Can you work these out from the model? Positions are in its coordinate system, mm. Face numbers are marked on the shaded views. A direction names the side the tool comes from. Round coordinates to 2 decimals unless told otherwise and drop trailing zeros. Order: outer loops, then holes, each group sorted by start corner. A loop starts at its lowest first (then second) coordinate and runs counter-clockwise, first axis right, second up. Notation, with made-up numbers: M 77,19.25 L 94,19.25 A16 cw 94,38.25 Z; hole C 70,-13.5 d8. An arc over 180 degrees is marked long. One line per question, with ' | ' between items.
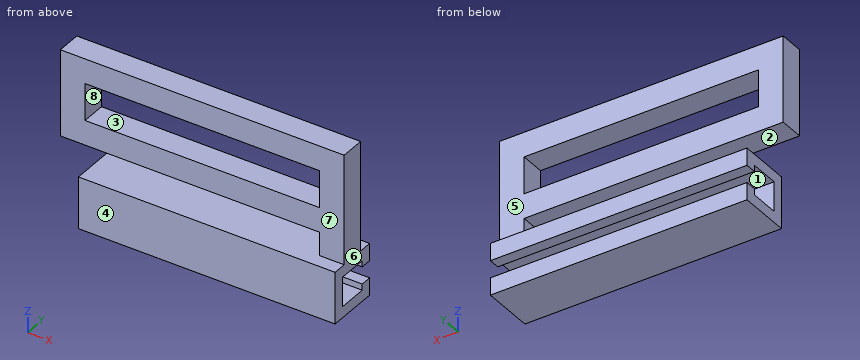
```python
from build123d import *

# Parameters (mm, degrees)
ESBO_O1_W                = 19
ESBO_O1_H                = 3
RESSALTO_EXTRUS_O1_DEPTH = 2
ESBO_O3_W                = 2.338389472
ESBO_O3_H                = 3.565642473
CORTE_EXTRUS_O2_DEPTH    = 3
ESBO_O4_W                = 4.2
ESBO_O4_H                = 4.2
ESBO_O4_W_2              = 2.2
ESBO_O4_H_2              = 2.2
RESSALTO_EXTRUS_O2_DEPTH = 21
ESBO_O5_W                = 2
ESBO_O5_H                = 2
CORTE_EXTRUS_O3_DEPTH    = 29
ESBO_O6_W                = 10.73629406
ESBO_O6_H                = 11.045994849
CORTE_EXTRUS_O4_DEPTH    = 4.5
CORTE_EXTRUS_O5_DEPTH    = 24


with BuildPart() as part:
    # Esboço1 → Ressalto-extrusão1 (new body)
    with BuildSketch(Plane(origin=(0, 0, 0), x_dir=(1, 0, 0), z_dir=(0, 1, 0))):
        Polygon((-10.479474548, 11.375), (12.520525452, 11.375), (12.520525452, -0.625), (10.520525452, -0.625), (-10.479474548, -0.625), (-10.479474548, 6.375), (10.520525452, 6.375), (10.520525452, 9.375), (-10.479474548, 9.375), align=None)
        with Locations((1.020525452, 2.875)):
            Rectangle(ESBO_O1_W, ESBO_O1_H, mode=Mode.SUBTRACT)
    extrude(amount=RESSALTO_EXTRUS_O1_DEPTH)

    # Esboço3 → Corte-extrusão2 (cut)
    with BuildSketch(Plane(origin=(0, 0, 0), x_dir=(1, 0, 0), z_dir=(0, 1, 0))):
        with Locations((-9.648669284, 10.261118249)):
            Rectangle(ESBO_O3_W, ESBO_O3_H)
    extrude(amount=CORTE_EXTRUS_O2_DEPTH, mode=Mode.SUBTRACT)

    # Esboço4 → Ressalto-extrusão2 (add)
    with BuildSketch(Plane.ZY.offset(8.479474548)):
        with Locations((-10.375, 1)):
            Rectangle(ESBO_O4_W, ESBO_O4_H)
        with Locations((-10.375, 1)):
            Rectangle(ESBO_O4_W_2, ESBO_O4_H_2, mode=Mode.SUBTRACT)
    extrude(amount=-RESSALTO_EXTRUS_O2_DEPTH)

    # Esboço5 → Corte-extrusão3 (cut)
    with BuildSketch(Plane.ZY.offset(8.479474548)):
        with Locations((-10.375, 1)):
            Rectangle(ESBO_O5_W, ESBO_O5_H)
    extrude(amount=-CORTE_EXTRUS_O3_DEPTH, mode=Mode.SUBTRACT)

    # Esboço6 → Corte-extrusão4 (cut, symmetric)
    with BuildSketch(Plane(origin=(0, 0, 0), x_dir=(1, 0, 0), z_dir=(0, 1, 0))):
        with Locations((-13.647621578, 13.152356314)):
            Rectangle(ESBO_O6_W, ESBO_O6_H)
    extrude(amount=CORTE_EXTRUS_O4_DEPTH, both=True, mode=Mode.SUBTRACT)

    # Esboço7 → Corte-extrusão5 (cut)
    with BuildSketch(Plane.ZY.offset(8.279474548)):
        Polygon((-11.075, 2.2), (-11.075, 3.370047827), (-9.675, 3.370047827), (-9.675, 2.2), (-9.175, 2.2), (-9.175, -0.2), (-11.575, -0.2), (-11.575, 2.2), align=None)
    extrude(amount=-CORTE_EXTRUS_O5_DEPTH, mode=Mode.SUBTRACT)


solid = part.part
```
(1) If we section it at D-D on y = 2.5: Please give me the cut outline in (x, z) (3 decimals), plus the area to 3 significant figures.
Final values:
outline: M -8.279,-12.475 L 12.521,-12.475 L 12.521,-11.075 L -8.279,-11.075 Z; M -8.279,-9.675 L 12.521,-9.675 L 12.521,-8.275 L -8.279,-8.275 Z | area: 58.2 mm^2
(2) On a 3-axis mill with a long thin cutter (end or side, diameter ignored), from which of +Z, -Z, +X, -X, +Y, -Y can I reach the whole of each face in a straight line? I mean the marked faces 1, 2, 3, 4 and 5. Say none if no direction works.
Final values:
face 1: +X, -X | face 2: -X, +Y, -Y | face 3: +Y, -Y | face 4: +Z, -Z, +X, -X, -Y | face 5: +Z, +X, -X, +Y
(3) If we section it at A-A on y = 1.55: Please give me the cut outline in (x, z) (3 decimals), plus the area to 3 significant figures.
Final values:
outline: M -10.479,-6.375 L 10.521,-6.375 L 10.521,-8.275 L -8.279,-8.275 L -8.279,-9.175 L 12.521,-9.175 L 12.521,0.625 L -10.479,0.625 Z; M -8.279,-12.475 L 12.521,-12.475 L 12.521,-11.575 L -8.279,-11.575 Z; hole M -8.479,-4.375 L 10.521,-4.375 L 10.521,-1.375 L -8.479,-1.375 Z | area: 145 mm^2
(4) If we section it at C-C on z = -2.75: Please give me the cut outline in (x, y), plus the area to 3 significant figures.
Final values:
outline: M -10.48,0 L -8.48,0 L -8.48,2 L -10.48,2 Z; M 10.52,0 L 12.52,0 L 12.52,2 L 10.52,2 Z | area: 8.00 mm^2
(5) Please list where these lines run through material, in increasing order: probe 1 along Z at (x, y) = (6.25, 1.2) (3 decimals); probe 2 along Y at (x, z) = (5.5, -11.25); probe 3 along Z at (x, y) = (9, 2.1) (3 decimals). Write a range as [from, to].
Final values:
probe 1: [-12.475, -11.575], [-9.175, -8.275], [-6.375, -4.375], [-1.375, 0.625] | probe 2: [-1.1, -0.2], [2.2, 3.1] | probe 3: [-12.475, -11.575], [-9.175, -8.275]
(6) Thinking about a two-plate mould opening in X: for the marked faces 6, 7 and 8, which applies, released by +X, released by -X, zero draft, split by the parting line, or undercut?
Final values:
face 6: released by +X | face 7: zero draft | face 8: undercut
(7) If we section it at B-B on x = -5.25: Please give me the cut outline in (y, z) (3 decimals), plus the area to 3 significant figures.
Final values:
outline: M -1.1,-12.475 L 3.1,-12.475 L 3.1,-11.075 L 2.2,-11.075 L 2.2,-11.575 L -0.2,-11.575 L -0.2,-9.175 L 2.2,-9.175 L 2.2,-9.675 L 3.1,-9.675 L 3.1,-8.275 L -1.1,-8.275 Z; M 0,-6.375 L 2,-6.375 L 2,-4.375 L 0,-4.375 Z; M 0,-1.375 L 2,-1.375 L 2,0.625 L 0,0.625 Z | area: 18.6 mm^2
(8) Will these pins go through, and if not, where does the flat tip stop? pin 1 Ø7 at (x, z) = (-0.5, -3.5) entering from +Y; pin 2 Ø7 at (x, z) = (1, -4) entering from -Y; pin 3 Ø2 at (y, z) = (0.5, -7.5) entering from -X.
Final values:
pin 1: y = 2 | pin 2: y = 0 | pin 3: x = -8.28
